The listing builds one solid part. Answer for the finished solid, in the listing's coordinates (mm). A direction names the side the tool comes from. Give positions to 0.01 mm unless a question says otherwise; leave off trailing zeros. Order: outer loops, then holes, each group sorted by start corner. A loop starts at its lowest first (then second) coordinate and runs counter-clockwise, first axis right, second up. Notation, with made-up numbers: (35, -15.75) - (64, -15.75) arc R30 ccw to (64, 12.25) - close; hole circle Ø2 at (74, 83.5). An arc over 180 degrees is marked (long way). Answer in a Markdown table with one row per item. Add a question column.
```python
from build123d import *

# Parameters (mm, degrees)
SKETCH1_W           = 10
SKETCH1_H           = 110
SKETCH1_W_2         = 15
SKETCH1_H_2         = 7.182689318
BOSS_EXTRUDE1_DEPTH = 10
SKETCH2_W           = 25
SKETCH2_H           = 7.182689318
BOSS_EXTRUDE2_DEPTH = 20
SKETCH3_R           = 2
CUT_EXTRUDE1_DEPTH  = 20
SKETCH4_R           = 2
CUT_EXTRUDE2_DEPTH  = 2
FILLET2_R           = 5
CHAMFER2_SIZE       = 5
FILLET3_R           = 6


with BuildPart() as part:
    # Sketch1 → Boss-Extrude1 (new body)
    with BuildSketch(Plane(origin=(0, 0, 0), x_dir=(1, 0, 0), z_dir=(0, 1, 0))):
        Polygon((-10, 110), (0, 110), (0, 121.590602055), (-90, 121.590602055), (-90, 110), align=None)
        with Locations((-5, 55)):
            Rectangle(SKETCH1_W, SKETCH1_H)
        with Locations((7.5, 3.591344659)):
            Rectangle(SKETCH1_W_2, SKETCH1_H_2)
    extrude(amount=BOSS_EXTRUDE1_DEPTH)

    # Sketch2 → Boss-Extrude2 (add)
    with BuildSketch(Plane.XZ):
        with Locations((2.5, -3.591344659)):
            Rectangle(SKETCH2_W, SKETCH2_H)
    extrude(amount=BOSS_EXTRUDE2_DEPTH)

    # Sketch3 → Cut-Extrude1 (cut)
    with BuildSketch(Plane(origin=(0, 0, -7.182689318), x_dir=(-1, 0, 0), z_dir=(0, 0, -1))):
        with Locations((-10, 2.5)):
            Circle(SKETCH3_R)
        with Locations(Location((-10, -12.5, 0), (0, 0, 180))):
            Circle(SKETCH3_R)
        with Locations((5, -12.5)):
            Circle(SKETCH3_R)
    extrude(amount=-CUT_EXTRUDE1_DEPTH, mode=Mode.SUBTRACT)

    # Sketch4 → Cut-Extrude2 (cut)
    with BuildSketch(Plane(origin=(0, 0, -7.182689318), x_dir=(-1, 0, 0), z_dir=(0, 0, -1))):
        Polygon((10, 0), (0, 0), (0, 10), (-15, 10), (-15, -20), (10, -20), align=None)
        with Locations((5, -12.5)):
            Circle(SKETCH4_R, mode=Mode.SUBTRACT)
        with Locations((-10, -12.5)):
            Circle(SKETCH4_R, mode=Mode.SUBTRACT)
        with Locations((-10, 2.5)):
            Circle(SKETCH4_R, mode=Mode.SUBTRACT)
    extrude(amount=-CUT_EXTRUDE2_DEPTH, mode=Mode.SUBTRACT)

    # Fillet2
    fillet2_edges = [part.edges().sort_by_distance(p)[0] for p in [
        (0, 5, -5.182689318),
        (-5, 0, -5.182689318),
    ]]
    fillet(fillet2_edges, radius=FILLET2_R)

    # Chamfer2
    chamfer2_edges = [part.edges().sort_by_distance(p)[0] for p in [
        (-50, 0, -110),
    ]]
    chamfer(chamfer2_edges, length=CHAMFER2_SIZE)

    # Fillet3
    fillet3_edges = [part.edges().sort_by_distance(p)[0] for p in [
        (0, 5, -121.590602055),
    ]]
    fillet(fillet3_edges, radius=FILLET3_R)


solid = part.part
```
(1) Each of these flat-tipped pins is pushed along its axis until it touches: P1, Ø3.5, axis at x = 10, y = 2.5, coming from the +Z side; P2, Ø4, axis at x = -45.5, y = 8.5, coming from the +Z side; P3, Ø3, axis at y = 5.5, z = -104, coming from the -X side; P4, Ø4, axis at x = -1, z = -43.5, coming from the -Y side. Where does it stop, or does it pass through?
(2) Straight lines are drawn through the part: line 1 (Y direction, x = 10, z = -3.6); line 2 (Z direction, x = -60, y = 6); line 3 (X direction, y = 0.25, z = -85). For each, find the intervals that lie inside material, in ascending order.
(3) Find section A-A, the plane y = 2.5. Write down the section's boundary in (x, z), plus the area to 3 significant figures.
(4) Find section B-B, the plane x = 10. Write down the section's boundary in (y, z).
(5) Find section D-D, the plane z = -31.5. Write down the section's boundary in (x, y).
(6) The mould has two halves that part along Y. Classify faces 1 (the face through (2, -5, 0)), 2 (the face through (-7, 10, -88)), 3 (the face through (-3.526, -11.148, -2.628)): +Y half, -Y half, draft (parallel to the pull), parting line (faces both ways), or undercut.
(7) For faces 4 (the face through (-9, 0, -87)), 5 (the face through (-51, 7, -110)), 6 (the face through (0, 5, -62)), determine the directions among +Z, -Z, +X, -X, +Y, -Y from which every point of the face is accessible in a straight line to the end or side of a thin tool.
(8) Find section C-C, the plane y = -12.5. Write down the section's boundary in (x, z).
Answer key:
| question | item | result |
|---|---|---|
| 1 | P1 | through |
| 1 | P2 | z = -110 |
| 1 | P3 | x = -10 |
| 1 | P4 | y = 0 |
| 2 | line 1 | -20 to -14.5, -10.5 to 0.5, 4.5 to 10 |
| 2 | line 2 | -121.59 to -110 |
| 2 | line 3 | -10 to 0 |
| 3 | outline | (-90, -121.59) - (-6, -121.59) arc R6 ccw to (0, -115.59) - (0, -10.18) arc R5 cw to (5, -5.18) - (8, -5.18) - (8, 0) - (-10, 0) - (-10, -112.5) - (-90, -112.5) - close; (12, -5.18) - (15, -5.18) - (15, 0) - (12, 0) - close |
| 3 | area | 2,000 mm² |
| 4 | outline | (-20, -5.18) - (-14.5, -5.18) - (-14.5, 0) - (-20, 0) - close; (-10.5, -5.18) - (0.5, -5.18) - (0.5, 0) - (-10.5, 0) - close; (4.5, -5.18) - (10, -5.18) - (10, 0) - (4.5, 0) - close |
| 5 | outline | (-10, 0) - (0, 0) - (0, 10) - (-10, 10) - close |
| 6 | face 1 | draft |
| 6 | face 2 | +Y half |
| 6 | face 3 | undercut |
| 7 | face 4 | -Z, +X, -X, -Y |
| 7 | face 5 | +Z, -X, +Y, -Y |
| 7 | face 6 | -Z, +X, +Y, -Y |
| 8 | outline | (-10, -5.18) - (-7, -5.18) - (-7, 0) - (-10, 0) - close; (-3, -5.18) - (8, -5.18) - (8, 0) - (-3, 0) - close; (12, -5.18) - (15, -5.18) - (15, 0) - (12, 0) - close |
